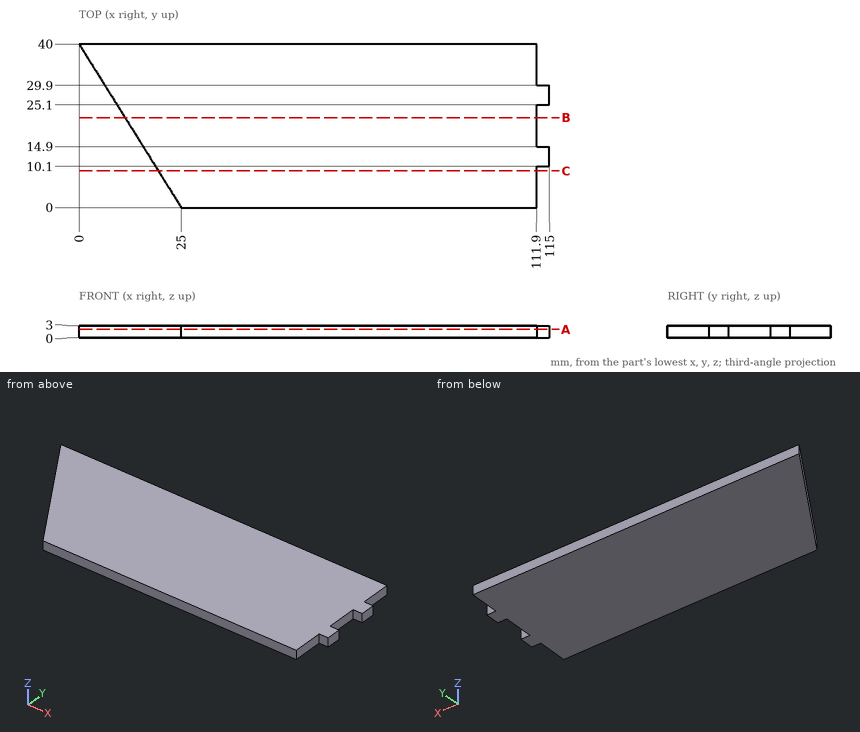
Could you check a few things on this drawing? It's one solid part, dimensions in mm from its lowest x, y, z. Coordinates: 2 decimals unless noted, no trailing zeros. Order: outer loops, then holes, each group sorted by start corner. A loop starts at its lowest first (then second) coordinate and runs counter-clockwise, first axis right, second up. Notation, with made-up numbers: (3.5, 62.25) - (21.5, 62.25) arc R19 ccw to (21.5, 80.25) - close; hole circle Ø10 at (13.25, 27.5). An arc over 180 degrees is marked (long way). Answer as a JSON object with one key per item and string values. Group by question number.
Q1. I need wall thicknesses on line 1 (X direction, y = 30.5, z = 1.35); line 2 (X direction, y = 12.5, z = 0.6); line 3 (Y direction, x = 16.5, z = 0.7). Which ranges of each line are inside material? Lowest first, please. Write a range as from..to.
Q2. Imagine slicing it at A-A (z = 2.05). Please give me the cut outline in (x, y), and give its area (3 significant figures).
Q3. Imagine slicing it at C-C (y = 9). Please give me the cut outline in (x, z) (3 decimals).
Q4. Imagine slicing it at B-B (y = 22). Please give me the cut outline in (x, z).
Q5. Will these pins go through, and if not, where does the flat tip stop? P1, Ø1.5, axis at y = 33, z = 1, coming from the +X side; P2, Ø0.9, axis at x = 113.5, z = 1.5, coming from the -Y side; P3, Ø0.9, axis at x = 113, z = 1.5, coming from the +Y side.
Determined:
{
 "1": {"line 1": "x = 5.94..111.9", "line 2": "x = 17.19..115", "line 3": "y = 13.6..40"},
 "2": {"outline": "(0, 40) - (25, 0) - (111.9, 0) - (111.9, 10.1) - (115, 10.1) - (115, 14.9) - (111.9, 14.9) - (111.9, 25.1) - (115, 25.1) - (115, 29.9) - (111.9, 29.9) - (111.9, 40) - close", "area": "4,010 mm2"},
 "3": {"outline": "(19.375, 0) - (111.9, 0) - (111.9, 3) - (19.375, 3) - close"},
 "4": {"outline": "(11.25, 0) - (111.9, 0) - (111.9, 3) - (11.25, 3) - close"},
 "5": {"P1": "stops at x = 111.9", "P2": "stops at y = 10.1", "P3": "stops at y = 29.9"}
}
